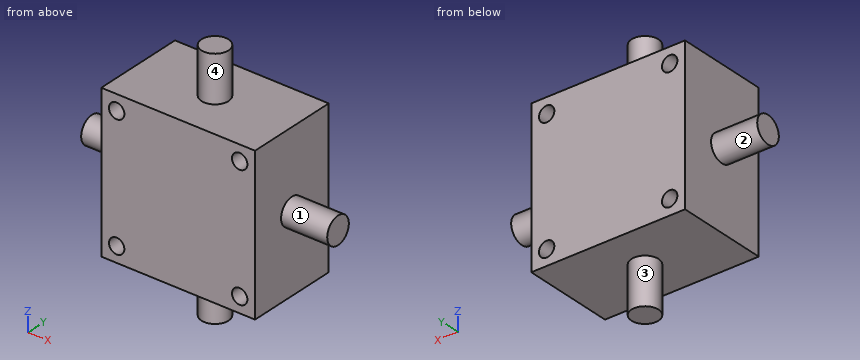
Autodesk Inventor part; units mm, degrees
ref_plane "YZ Plane" through (0, 0, 0) normal (1, 0, 0) x (0, 1, 0)
ref_plane "XZ Plane" through (0, 0, 0) normal (0, 1, 0) x (-1, 0, 0)
ref_plane "XY Plane" through (0, 0, 0) normal (0, 0, 1) x (1, 0, 0)
sketch "Sketch1" plane through (0, 0, 0) normal (0, 1, 0) x (-1, 0, 0)
  line L0 (-15.875, -15.875) -> (15.875, -15.875)
  line L1 (15.875, -15.875) -> (15.875, 15.875)
  line L2 (15.875, 15.875) -> (-15.875, 15.875)
  line L3 (-15.875, 15.875) -> (-15.875, -15.875)
  line L4 (-15.875, -15.875) -> (15.875, 15.875) construction
  line L5 (15.875, -15.875) -> (-15.875, 15.875) construction
  point P0 (0, 0)
  dimension "d0" = 31.75
  dimension "d1" = 31.75
extrude "Extrusion1" add sketch "Sketch1" along normal mid plane 19.05
sketch "Sketch2" plane through (0, 9.525, 0) normal (0, 1, 0) x (1, 0, 0)
  circle A0 centre (-12.7, -12.7) radius 1.5875
  circle A1 centre (-12.7, 12.7) radius 1.5875
  circle A2 centre (12.7, -12.7) radius 1.5875
  circle A3 centre (12.7, 12.7) radius 1.5875
  point P0 (0, 0)
  dimension "d4" = 3.175
  dimension "d5" = 3.175
  dimension "d6" = 3.175
  dimension "d7" = 3.175
extrude "Extrusion2" cut sketch "Sketch2" against normal through all
sketch "Sketch3" plane through (-15.875, 9.525, 15.875) normal (0, 0, 1) x (1, 0, 0)
  circle A0 centre (15.875, -9.525) radius 2.794
  dimension "d10" = 5.588
sketch "Sketch4" plane through (15.875, -9.525, -15.875) normal (1, 0, 0) x (0, 0, -1)
  circle A0 centre (-15.875, 9.525) radius 2.794
  dimension "d11" = 5.588
sketch "Sketch5" plane through (15.875, 9.525, -15.875) normal (0, 0, -1) x (-1, 0, 0)
  circle A0 centre (15.875, -9.525) radius 2.794
  dimension "d12" = 5.588
sketch "Sketch6" plane through (-15.875, -9.525, 15.875) normal (-1, 0, 0) x (0, 0, 1)
  circle A0 centre (-15.875, 9.525) radius 2.794
  dimension "d13" = 5.588
extrude "Extrusion3" add sketch "Sketch6" along normal blind 9.525
extrude "Extrusion4" add sketch "Sketch5" along normal blind 9.525
extrude "Extrusion5" add sketch "Sketch4" along normal blind 9.525
extrude "Extrusion6" add sketch "Sketch3" along normal blind 9.525
properties part number "ZFSWHA-1-20+_Switch"
The model under review builds one solid part; all positions refer to its coordinate system, in mm. Face numbers are marked on the shaded views. A direction names the side the tool comes from. Round coordinates to 2 decimals unless told otherwise and drop trailing zeros. Loops run counter-clockwise (first coordinate to the right, second up) from the corner with the lowest first, then second, coordinate; pieces in that order, holes last. Notation, with made-up numbers: (-14.5, 47.5) -> (31.5, 47.5) arc R31 ccw to (31.5, 81.5) -> close; hole circle Ø7 at (-18.5, 61). An arc over 180 degrees is marked (long way). Answer as a JSON object with one key per item and string values. Group by question number.
1) For line 1 (Z direction, x = 12.7, y = -3) (1 decimal); line 2 (Z direction, x = 16, y = 0.25), list the stretches that pass through material, from the lowest coordinate up. Write a range as [from, to].
2) We need section A-A on x = 12.7. Write out the cut boundary in (y, z) (1 decimal).
3) For the marked faces 1, 2, 3 and 4, list the 3-axis set-ups (+Z, -Z, +X, -X, +Y, -Y) from which the entire face can be reached by the end or side of a thin tool; tool diameter is ignored.
4) We need section C-C on y = 0. Write out the cut boundary in (x, z) (1 decimal).
5) We need section B-B on z = -12.7. Write out the cut boundary in (x, y) (1 decimal).
6) We need section D-D on z = -0.5. Write out the cut boundary in (x, y) (3 decimals), then the cut area to 3 significant figures.
7) For pin 1 Ø4 at (x, z) = (9, 16.5) entering from +Y (3 decimals); pin 2 Ø4 at (x, y) = (13.5, 5.5) entering from +Z (3 decimals); pin 3 Ø3 at (x, z) = (-12.7, -12.7) entering from -Y; pin 4 Ø5 at (y, z) = (-2, -6) entering from -X (3 decimals), all flat-tipped, find the tip position at first contact; note any pin that passes through.
Result set:
{
 "1": {"line 1": "[-15.9, -14.3], [-11.1, 11.1], [14.3, 15.9]", "line 2": "[-2.78, 2.78]"},
 "2": {"outline": "(-9.5, -15.9) -> (9.5, -15.9) -> (9.5, -14.3) -> (-9.5, -14.3) -> close; (-9.5, -11.1) -> (9.5, -11.1) -> (9.5, 11.1) -> (-9.5, 11.1) -> close; (-9.5, 14.3) -> (9.5, 14.3) -> (9.5, 15.9) -> (-9.5, 15.9) -> close"},
 "3": {"face 1": "+X", "face 2": "-X", "face 3": "-Z", "face 4": "+Z"},
 "4": {"outline": "(-25.4, -2.8) -> (-15.9, -2.8) -> (-15.9, -15.9) -> (-2.8, -15.9) -> (-2.8, -25.4) -> (2.8, -25.4) -> (2.8, -15.9) -> (15.9, -15.9) -> (15.9, -2.8) -> (25.4, -2.8) -> (25.4, 2.8) -> (15.9, 2.8) -> (15.9, 15.9) -> (2.8, 15.9) -> (2.8, 25.4) -> (-2.8, 25.4) -> (-2.8, 15.9) -> (-15.9, 15.9) -> (-15.9, 2.8) -> (-25.4, 2.8) -> close; hole circle Ø3.2 at (-12.7, -12.7); hole circle Ø3.2 at (-12.7, 12.7); hole circle Ø3.2 at (12.7, -12.7); hole circle Ø3.2 at (12.7, 12.7)"},
 "5": {"outline": "(-15.9, -9.5) -> (-14.3, -9.5) -> (-14.3, 9.5) -> (-15.9, 9.5) -> close; (-11.1, -9.5) -> (11.1, -9.5) -> (11.1, 9.5) -> (-11.1, 9.5) -> close; (14.3, -9.5) -> (15.9, -9.5) -> (15.9, 9.5) -> (14.3, 9.5) -> close"},
 "6": {"outline": "(-25.4, -2.749) -> (-15.875, -2.749) -> (-15.875, -9.525) -> (15.875, -9.525) -> (15.875, -2.749) -> (25.4, -2.749) -> (25.4, 2.749) -> (15.875, 2.749) -> (15.875, 9.525) -> (-15.875, 9.525) -> (-15.875, 2.749) -> (-25.4, 2.749) -> close", "area": "710 mm²"},
 "7": {"pin 1": "y = 9.525", "pin 2": "z = 15.875", "pin 3": "through", "pin 4": "x = -15.875"}
}
